from build123d import *

# Parameters (mm, degrees)
F0_W     = 76.2
F0_H     = 38.1
F0_R     = 4.06875
F0_R_2   = 3.175
F1_DEPTH = 5
F2_W     = 4
F2_H     = 19.05
F3_DEPTH = 19.05
F4_W     = 3
F4_H     = 15.875
F5_DEPTH = 12.7
F7_DEPTH = 4
F8_R     = 1.349997
F9_DEPTH = 3


with BuildPart() as f1:
    # F0 (on Top) → F1 (new body)
    with BuildSketch(Plane.XY):
        with Locations((38.1, 0)):
            Rectangle(F0_W, F0_H)
        with Locations((63.5, 0)):
            Circle(F0_R, mode=Mode.SUBTRACT)
        with Locations((50.8, 9.525)):
            Circle(F0_R_2, mode=Mode.SUBTRACT)
        with Locations((-38.1, 0)):
            Rectangle(F0_W, F0_H)
        with Locations((-63.5, 0)):
            Circle(F0_R, mode=Mode.SUBTRACT)
        with Locations((-50.8, 9.525)):
            Circle(F0_R_2, mode=Mode.SUBTRACT)
    extrude(amount=F1_DEPTH)

    # F2 (on face) → F3 (join)
    with BuildSketch(Plane.XY.offset(5)):
        with Locations((-11.89, 9.525)):
            Rectangle(F2_W, F2_H)
        with Locations((-11.89, -9.525)):
            Rectangle(F2_W, F2_H)
    extrude(amount=F3_DEPTH)

    # F4 (on face) → F5 (join)
    with BuildSketch(Plane.XY.offset(5)):
        with Locations((-33.425, 4.7625)):
            Rectangle(F4_W, F4_H)
    extrude(amount=F5_DEPTH)

    # F6 (on face) → F7 (cut, through all)
    with BuildSketch(Plane.YZ.offset(-9.89)):
        with BuildLine():
            Line((-8.099996, 14.525), (-5.499996, 14.525))
            ThreePointArc((-5.499996, 14.525), (-8.099996, 17.125), (-10.699996, 14.525))
            Line((-10.699996, 14.525), (-8.099996, 14.525))
        make_face()
        with BuildLine():
            ThreePointArc((-10.699996, 14.525), (-8.099996, 11.925), (-5.499996, 14.525))
            Line((-5.499996, 14.525), (-8.099996, 14.525))
            Line((-8.099996, 14.525), (-10.699996, 14.525))
        make_face()
    extrude(amount=-F7_DEPTH, mode=Mode.SUBTRACT)

    # F8 (on face) → F9 (cut, through all)
    with BuildSketch(Plane(origin=(-34.925, 0, 0), x_dir=(0, -1, 0), z_dir=(-1, 0, 0))):
        with Locations((-9.787496, 12.949984)):
            Circle(F8_R)
        with Locations((0.262496, 12.949984)):
            Circle(F8_R)
    extrude(amount=-F9_DEPTH, mode=Mode.SUBTRACT)


solid = f1.part
Verification items for the finished model (mm, model axes). A direction names the side the tool comes from. Coordinates: 2 decimals unless noted, no trailing zeros. Order: outer loops, then holes, each group sorted by start corner. A loop starts at its lowest first (then second) coordinate and runs counter-clockwise, first axis right, second up.
Item 1: Section check A-A, the plane x = 63.5. Enter the section's corners in (y, z), then the cut area to 3 significant figures.
Filled in:
outline: (-19.05, 0) - (-4.07, 0) - (-4.07, 5) - (-19.05, 5) - close; (4.07, 0) - (19.05, 0) - (19.05, 5) - (4.07, 5) - close
area: 150 mm2
Item 2: Section check D-D, the plane z = 20.75. Enter the section's corners in (x, y).
Filled in:
outline: (-13.89, -19.05) - (-9.89, -19.05) - (-9.89, 19.05) - (-13.89, 19.05) - close
Item 3: Depth check by flat-ended pin: pin 1 (4 mm diameter, centred on y = 4.5, z = 11, fed in from +X); pin 2 (10 mm diameter, centred on x = 7.5, y = 5.5, fed in from +Z); pin 3 (5.5 mm diameter, centred on x = 50.8, y = 9.525, fed in from -Z); pin 4 (1.5 mm diameter, centred on x = -33.5, y = 7, fed in from +Z). Enter the tip coordinate at first touch or a pass-through.
Filled in:
pin 1: stops at x = -9.89
pin 2: stops at z = 5
pin 3: passes through
pin 4: stops at z = 17.7
Item 4: Release check for a two-part mould opening along Z. For faces 4 (the face through (33, 0, 5)), 5 (the face through (-9.89, 0, 14)), 6 (the face through (-33.446, 0.03, 11.632)) record: +Z half, -Z half, draft (parallel to the pull), parting line (faces both ways), or undercut.
Filled in:
face 4: +Z half
face 5: draft
face 6: undercut
Item 5: Section check C-C, the plane y = -8. Enter the section's corners in (x, z).
Filled in:
outline: (-76.2, 0) - (76.2, 0) - (76.2, 5) - (-9.89, 5) - (-9.89, 11.93) - (-13.89, 11.93) - (-13.89, 5) - (-76.2, 5) - close; (-13.89, 17.12) - (-9.89, 17.12) - (-9.89, 24.05) - (-13.89, 24.05) - close
Item 6: Section check B-B, the plane z = 7.25. Enter the section's corners in (x, y) (3 decimals), then the cut area to 3 significant figures.
Filled in:
outline: (-34.925, -3.175) - (-31.925, -3.175) - (-31.925, 12.7) - (-34.925, 12.7) - close; (-13.89, -19.05) - (-9.89, -19.05) - (-9.89, 19.05) - (-13.89, 19.05) - close
area: 200 mm2
Item 7: Access from +Z, -Z, +X, -X, +Y, -Y to the whole of each face (thin tool, end or side, straight path). Record for faces 1 (the face through (-33, 5, 17.7)), 2 (the face through (-33.45, 10.86, 12.13)), 3 (the face through (-33, 12.7, 11)).
Filled in:
face 1: +Z, -X, +Y, -Y
face 2: -X
face 3: +Z, -X, +Y
Item 8: Material ranges on L1, parallel to X at y = 2, z = 6.5 (3 decimals); L2, parallel to Y at x = -50.8, z = 1.35; L3, parallel to X at y = 12, z = 4, recorded low to high.
Filled in:
L1: x = -34.925 to -31.925, -13.89 to -9.89
L2: y = -19.05 to 6.35, 12.7 to 19.05
L3: x = -76.2 to -52.79, -48.81 to 48.81, 52.79 to 76.2
